Here's how the part is built. I have some questions about the finished solid (model axes, mm). A direction names the side the tool comes from. Round coordinates to 2 decimals unless told otherwise and drop trailing zeros. Loops run counter-clockwise (first coordinate to the right, second up) from the corner with the lowest first, then second, coordinate; pieces in that order, holes last. Notation, with made-up numbers: (81, 12) -> (93, 12) arc R21 ccw to (93, 49) -> close; hole circle Ø3 at (18.5, -9). An arc over 180 degrees is marked (long way). Use CSV: the item, a comma, the result in double quotes. Start each with the question number.
from build123d import *

# Parameters (mm, degrees)
SKETCH_1_R          = 10.25
EXTRUDE_2_DEPTH     = 0.5
FILLET_1_R          = 23
CUT_EXTRUDE_1_DEPTH = 55
FILLET_2_R          = 2
FILLET_3_R          = 5


with BuildPart() as part:
    # 草图1 → 凸台-拉伸2 (new body)
    with BuildSketch(Plane.XY):
        with BuildLine():
            ThreePointArc((-9.125563074, 59.5), (-35.197591975, 61.447591975), (-33.25, 35.375563074))
            Line((-33.25, 35.375563074), (-33.25, -35.375563074))
            ThreePointArc((-33.25, -35.375563074), (-35.197591975, -61.447591975), (-9.125563074, -59.5))
            Line((-9.125563074, -59.5), (9.125563074, -59.5))
            ThreePointArc((9.125563074, -59.5), (35.197591975, -61.447591975), (33.25, -35.375563074))
            Line((33.25, -35.375563074), (33.25, 35.375563074))
            ThreePointArc((33.25, 35.375563074), (35.197591975, 61.447591975), (9.125563074, 59.5))
            Line((9.125563074, 59.5), (-9.125563074, 59.5))
        make_face()
        with Locations((23, -49.25)):
            Circle(SKETCH_1_R, mode=Mode.SUBTRACT)
        with Locations((-23, -49.25)):
            Circle(SKETCH_1_R, mode=Mode.SUBTRACT)
        with Locations((23, 49.25)):
            Circle(SKETCH_1_R, mode=Mode.SUBTRACT)
        with Locations((-23, 49.25)):
            Circle(SKETCH_1_R, mode=Mode.SUBTRACT)
    extrude(amount=EXTRUDE_2_DEPTH)

    # 圆角1
    fillet_1_edges = [part.edges().sort_by_distance(p)[0] for p in [
        (33.25, -35.375563074, 0.25),
        (9.125563074, -59.5, 0.25),
        (-9.125563074, -59.5, 0.25),
        (-33.25, -35.375563074, 0.25),
        (-33.25, 35.375563074, 0.25),
        (-9.125563074, 59.5, 0.25),
        (9.125563074, 59.5, 0.25),
        (33.25, 35.375563074, 0.25),
    ]]
    fillet(fillet_1_edges, radius=FILLET_1_R)

    # 草图2 → 切除-拉伸1 (cut)
    with BuildSketch(Plane(origin=(0, 0, 0), x_dir=(-1, 0, 0), z_dir=(0, 0, -1))):
        Polygon((20, 33.37288914), (4.414691366, 0), (20, -33.37288914), align=None)
        Polygon((-11.170617268, 33.37288914), (0, 9.453197817), (11.170617268, 33.37288914), align=None)
        Polygon((-4.414691366, 0), (-20, 33.37288914), (-20, -33.37288914), align=None)
        Polygon((11.170617268, -33.37288914), (0, -9.453197817), (-11.170617268, -33.37288914), align=None)
    extrude(amount=-CUT_EXTRUDE_1_DEPTH, mode=Mode.SUBTRACT)

    # 圆角2
    fillet_2_edges = [part.edges().sort_by_distance(p)[0] for p in [
        (20, 33.37288914, 0.25),
        (20, -33.37288914, 0.25),
        (11.170617268, 33.37288914, 0.25),
        (-11.170617268, 33.37288914, 0.25),
        (11.170617268, -33.37288914, 0.25),
        (0, -9.453197817, 0.25),
        (-11.170617268, -33.37288914, 0.25),
        (-20, 33.37288914, 0.25),
        (-20, -33.37288914, 0.25),
    ]]
    fillet(fillet_2_edges, radius=FILLET_2_R)

    # 圆角3
    fillet_3_edges = [part.edges().sort_by_distance(p)[0] for p in [
        (4.414691366, 0, 0.25),
        (-4.414691366, 0, 0.25),
    ]]
    fillet(fillet_3_edges, radius=FILLET_3_R)


solid = part.part
Q1. I want a section at B-B, the plane y = -49.25. List the corners of the cut face in (x, z) for me.
Q2. If we mould it in two halves opening along X, with no side actions, what happens to faces 5 (the cylindrical face through (-34.245, -33.258, 0.254)), 6 (the flat face through (-1, 1, 0.5)), 7 (the flat face through (10.87, -13.82, 0.25))? For each: pulls with the +X half, pulls with the -X half, needs draft (parallel to the pull), parting line crosses it, or undercut.
Q3. I want a section at C-C, the plane z = 0.3. Count the separate pieces of the cut face and the enclosed holes in it, then the cut area to 3 significant figures.
Q4. I want a section at A-A, the plane x = -23. List the corners of the cut face in (y, z) for me.
Q5. I want a section at D-D, the plane y = 12. List the corners of the cut face in (x, z) for me.
Q6. Will this pin go through, and if not, where does the flat tip stop? pin 1 Ø6 at (x, y) = (20.5, 30.5) entering from -Z.
Q7. I need wall thicknesses on line 1 along Y through (x, z) = (-23, 0.35); line 2 along Y through (x, z) = (-20.5, 0.35); line 3 along X through (y, z) = (-57, 0.3). Which ranges of each line are inside material? Lowest first, please.
Q8. For faces 1 (the cylindrical face through (34.3, 33.44, 0.25)), 2 (the cylindrical face through (7.008, -60.495, 0.254)), 3 (the cylindrical face through (7.008, 60.495, 0.254)), 4 (the flat face through (-10.87, 13.82, 0.25)), which set-ups out of +Z, -Z, +X, -X, +Y, -Y let a thin tool reach every point of the face, with its end or its side?
Values found:
1,outline,"(-40.25, 0) -> (-33.25, 0) -> (-33.25, 0.5) -> (-40.25, 0.5) -> close; (-12.75, 0) -> (12.75, 0) -> (12.75, 0.5) -> (-12.75, 0.5) -> close; (33.25, 0) -> (40.25, 0) -> (40.25, 0.5) -> (33.25, 0.5) -> close"
2,face 5,"pulls with the -X half"
2,face 6,"needs draft"
2,face 7,"undercut"
3,separate pieces,"1"
3,enclosed holes,"8"
3,area,"6,200 mm2"
4,outline,"(-66.5, 0) -> (-59.5, 0) -> (-59.5, 0.5) -> (-66.5, 0.5) -> close; (-39, 0) -> (39, 0) -> (39, 0.5) -> (-39, 0.5) -> close; (59.5, 0) -> (66.5, 0) -> (66.5, 0.5) -> (59.5, 0.5) -> close"
5,outline,"(-33.25, 0) -> (-20, 0) -> (-20, 0.5) -> (-33.25, 0.5) -> close; (-10.02, 0) -> (-1.19, 0) -> (-1.19, 0.5) -> (-10.02, 0.5) -> close; (1.19, 0) -> (10.02, 0) -> (10.02, 0.5) -> (1.19, 0.5) -> close; (20, 0) -> (33.25, 0) -> (33.25, 0.5) -> (20, 0.5) -> close"
6,pin 1,"z = 0"
7,line 1,"-66.5 to -59.5, -39 to 39, 59.5 to 66.5"
7,line 2,"-66.32 to -59.19, -39.31 to 39.31, 59.19 to 66.32"
7,line 3,"-38.41 to -29.71, -16.29 to 16.29, 29.71 to 38.41"
8,face 1,"+Z, -Z, +X"
8,face 2,"+Z, -Z, -Y"
8,face 3,"+Z, -Z, +Y"
8,face 4,"+Z, -Z"
